from build123d import *

# Parameters (mm, degrees)
BOSS_EXTRUDE2_DEPTH      = 6
BOSS_EXTRUDE2_DEPTH_BACK = 6
SKETCH1_R                = 8.15
SKETCH2_R                = 2.6
CUT_EXTRUDE1_DEPTH       = 21.807991253


with BuildPart() as part:
    # Sketch1 → Boss-Extrude2 (new, two sides: drawn at the far end of the back side and taken through both)
    with BuildSketch(Plane.XY.offset(-BOSS_EXTRUDE2_DEPTH_BACK)):
        with BuildLine():
            Line((-5, 8.95), (5, 8.95))
            Line((5, 8.95), (5, 7.180703308))
            ThreePointArc((5, 7.180703308), (8.75, 0), (5, -7.180703308))
            Line((5, -7.180703308), (5, -8.95))
            Line((5, -8.95), (-5, -8.95))
            Line((-5, -8.95), (-5, -7.180703308))
            ThreePointArc((-5, -7.180703308), (-8.75, 0), (-5, 7.180703308))
            Line((-5, 7.180703308), (-5, 8.95))
        make_face()
        Circle(SKETCH1_R, mode=Mode.SUBTRACT)
    extrude(amount=BOSS_EXTRUDE2_DEPTH + BOSS_EXTRUDE2_DEPTH_BACK)

    # Sketch2 → Cut-Extrude1 (cut, through all)
    with BuildSketch(Plane(origin=(0, 8.95, 0), x_dir=(1, 0, 0), z_dir=(0, 1, 0))):
        with Locations(Location((0, 0, 0), (0, 0, 270))):
            Circle(SKETCH2_R)
    extrude(amount=-CUT_EXTRUDE1_DEPTH, mode=Mode.SUBTRACT)


solid = part.part
Read the model definition and answer for the solid it produces. Units are mm, in the model's axes. A direction names the side the tool comes from. Give positions to 0.01 mm unless a question says otherwise; leave off trailing zeros. Write each loop counter-clockwise with the first axis right and the second up, starting at its lowest first coordinate (ties: lowest second). Pieces come first, ordered by that corner, then holes. Notation, with made-up numbers: (57.5, -35) - (77.5, -35) arc R16 cw to (77.5, -13) - close; hole circle Ø1 at (51.5, 18.25). An arc over 180 degrees is marked (long way). Answer in a Markdown table with one row per item. Add a question column.
Item 1: Section B-B, the plane z = 0 is taken. Write down the section's boundary in (x, y), and give its area (3 significant figures).
Item 2: Determine the mould class of faces 1 (the face through (0.1, -8.5, -2.6)), 2 (the face through (0, 8.95, -3)), 3 (the face through (8, -3, 6)) for opening direction Z: pulls with the +Z half, pulls with the -Z half, needs draft (parallel to the pull), parting line crosses it, or undercut.
Item 3: Section A-A, the plane y = 0 is taken. Write down the section's boundary in (x, z).
Item 4: A tool of negligible diameter and unlimited length cuts with its end or side. For faces 4 (the face through (-5, -8, 0)), 5 (the face through (5, 8, 0)), 6 (the face through (-5, 8, 0)), 7 (the face through (5, -8, 0)), from which of +Z, -Z, +X, -X, +Y, -Y can it reach the whole face along a straight path? Write none if from no direction.
Item 5: Find the intervals of material crossed by L1, parallel to X at y = 8.55, z = 0; L2, parallel to Z at x = 0, y = -8.4; L3, parallel to Y at x = -7.5, z = 0.75, in increasing order.
Item 6: Section C-C, the plane x = 0 is taken. Write down the section's boundary in (y, z), and give its area (3 significant figures).
Item 7: Section D-D, the plane z = 4.75 is taken. Write down the section's boundary in (x, y), and give its area (3 significant figures).
Item 8: Flat-ended cylindrical pins translate along their axes: P1, Ø0.9, axis at y = -8.5, z = 0, coming from the +X side; P2, Ø3, axis at y = 3.5, z = -2.5, coming from the -X side; P3, Ø4, axis at y = 3, z = 0, coming from the +X side. Find the tip coordinate at first contact, or state that the pin passes through.
Recorded:
| question | item | result |
|---|---|---|
| 1 | outline | (-5, -8.95) - (-2.6, -8.95) - (-2.6, -7.72) arc R8.15 cw to (-2.6, 7.72) - (-2.6, 8.95) - (-5, 8.95) - (-5, 7.18) arc R8.75 ccw to (-5, -7.18) - close; (2.6, -8.95) - (5, -8.95) - (5, -7.18) arc R8.75 ccw to (5, 7.18) - (5, 8.95) - (2.6, 8.95) - (2.6, 7.72) arc R8.15 cw to (2.6, -7.72) - close |
| 1 | area | 36.1 mm2 |
| 2 | face 1 | undercut |
| 2 | face 2 | needs draft |
| 2 | face 3 | pulls with the +Z half |
| 3 | outline | (-8.75, -6) - (-8.15, -6) - (-8.15, 6) - (-8.75, 6) - close; (8.15, -6) - (8.75, -6) - (8.75, 6) - (8.15, 6) - close |
| 4 | face 4 | +Z, -Z, -X, -Y |
| 4 | face 5 | +Z, -Z, +X, +Y |
| 4 | face 6 | +Z, -Z, -X, +Y |
| 4 | face 7 | +Z, -Z, +X, -Y |
| 5 | L1 | x = -5 to -2.6, 2.6 to 5 |
| 5 | L2 | z = -6 to -2.6, 2.6 to 6 |
| 5 | L3 | y = -4.51 to -3.19, 3.19 to 4.51 |
| 6 | outline | (-8.95, -6) - (-8.15, -6) - (-8.15, -2.6) - (-8.95, -2.6) - close; (-8.95, 2.6) - (-8.15, 2.6) - (-8.15, 6) - (-8.95, 6) - close; (8.15, -6) - (8.95, -6) - (8.95, -2.6) - (8.15, -2.6) - close; (8.15, 2.6) - (8.95, 2.6) - (8.95, 6) - (8.15, 6) - close |
| 6 | area | 10.9 mm2 |
| 7 | outline | (-5, -8.95) - (5, -8.95) - (5, -7.18) arc R8.75 ccw to (5, 7.18) - (5, 8.95) - (-5, 8.95) - (-5, 7.18) arc R8.75 ccw to (-5, -7.18) - close; hole circle Ø16.3 at (0, 0) |
| 7 | area | 45.9 mm2 |
| 8 | P1 | stops at x = 5 |
| 8 | P2 | stops at x = -8.52 |
| 8 | P3 | stops at x = 8.69 |
